The listing builds one solid part. Answer for the finished solid, in the listing's coordinates (mm). Face numbers are marked on the shaded views. A direction names the side the tool comes from. Give positions to 0.01 mm unless a question says otherwise; leave off trailing zeros. Order: outer loops, then holes, each group sorted by start corner. A loop starts at its lowest first (then second) coordinate and runs counter-clockwise, first axis right, second up. Notation, with made-up numbers: (74.5, 38.25) - (126.5, 38.25) arc R27 cw to (126.5, 65.25) - close; hole circle Ø11 at (89.5, -29.5). An arc over 180 degrees is marked (long way). Answer as a JSON object with one key per item and string values. Group by question number.
Q1. A cutting plane is placed at A-A, the plane x = 72.5. Give the vertices of the cut face in (y, z), and give its area (3 significant figures).
Q2. A cutting plane is placed at B-B, the plane x = 31. Give the vertices of the cut face in (y, z).
Q3. Consider line 1 (Y direction, x = 2.5, z = 1.1); line 2 (Y direction, x = 47, z = 5.5); line 3 (Z direction, x = 6.5, y = 10.75). Determine where each line is inside the solid, lowest interval first.
Q4. For the marked faces 1, 2 and 3, determine the directions among +Z, -Z, +X, -X, +Y, -Y from which every point of the face is accessible in a straight line to the end or side of a thin tool.
Q5. A cutting plane is placed at D-D, the plane y = 4.75. Give the vertices of the cut face in (x, z), and give its area (3 significant figures).
Q6. Given pin 1 (5 mm diameter, centred on x = 56, y = 2, fed in from +Z); pin 2 (3 mm diameter, centred on y = 8.5, z = 10.5, fed in from +X); pin 3 (1.8 mm diameter, centred on y = 10, z = 7.5, fed in from -X), each flat-ended and moving along its own axis, determine where each tip first touches the part or whether it passes through.
from build123d import *

# Parameters (mm, degrees)
SKETCH1_W           = 75
SKETCH1_H           = 12.8
BOSS_EXTRUDE1_DEPTH = 3.4
SKETCH2_W           = 28.4
SKETCH2_H           = 3.5
BOSS_EXTRUDE2_DEPTH = 12
SKETCH2_3_R         = 1
SKETCH2_3_R_2       = 1.000959723
CUT_EXTRUDE1_DEPTH  = 12


with BuildPart() as part:
    # Sketch1 → Boss-Extrude1 (new body)
    with BuildSketch(Plane.XY):
        with Locations((37.5, 6.4)):
            Rectangle(SKETCH1_W, SKETCH1_H)
    extrude(amount=BOSS_EXTRUDE1_DEPTH)

    # Sketch2 → Boss-Extrude2 (add)
    with BuildSketch(Plane.XY.offset(3.4)):
        with Locations((33.2, 9.05)):
            Rectangle(SKETCH2_W, SKETCH2_H)
    extrude(amount=BOSS_EXTRUDE2_DEPTH)

    # Sketch2_3 → Cut-Extrude1 (cut)
    with BuildSketch(Plane.XY.offset(3.4)):
        with Locations((72.5, 10.3)):
            Circle(SKETCH2_3_R)
        with Locations((2.5, 10.3)):
            Circle(SKETCH2_3_R_2)
    extrude(amount=-CUT_EXTRUDE1_DEPTH, mode=Mode.SUBTRACT)


solid = part.part
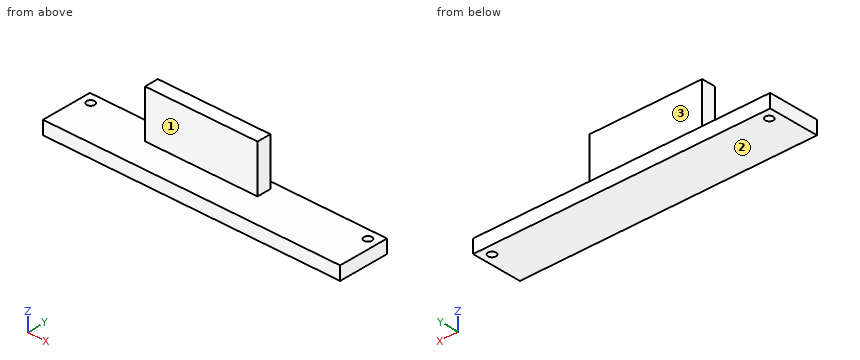
Reply:
{
 "1": {"outline": "(0, 0) - (9.3, 0) - (9.3, 3.4) - (0, 3.4) - close; (11.3, 0) - (12.8, 0) - (12.8, 3.4) - (11.3, 3.4) - close", "area": "36.7 mm^2"},
 "2": {"outline": "(0, 0) - (12.8, 0) - (12.8, 3.4) - (10.8, 3.4) - (10.8, 15.4) - (7.3, 15.4) - (7.3, 3.4) - (0, 3.4) - close"},
 "3": {"line 1": "y = 0 to 9.3, 11.3 to 12.8", "line 2": "y = 7.3 to 10.8", "line 3": "z = 0 to 3.4"},
 "4": {"face 1": "+Z, +X, -X, -Y", "face 2": "-Z, +X, -X, +Y, -Y", "face 3": "+Z, +X, -X, +Y"},
 "5": {"outline": "(0, 0) - (75, 0) - (75, 3.4) - (0, 3.4) - close", "area": "255 mm^2"},
 "6": {"pin 1": "stops at z = 3.4", "pin 2": "stops at x = 47.4", "pin 3": "stops at x = 19"}
}
